The listing builds one solid part. Answer for the finished solid, in the listing's coordinates (mm). A direction names the side the tool comes from. Coordinates: 2 decimals unless noted, no trailing zeros. Loops run counter-clockwise (first coordinate to the right, second up) from the corner with the lowest first, then second, coordinate; pieces in that order, holes last. Notation, with made-up numbers: M -15.75,34 L 43.25,34 A27 cw 43.25,65 Z; hole C -35,84.5 d2. An arc over 180 degrees is marked long. Answer as a JSON object with one key per item and string values. Group by question number.
1. A cutting plane is placed at A-A on z = 62. Give the vertices of the cut face in (x, y).
2. Straight lines are drawn through the part: L1, parallel to X at y = -65, z = 36; L2, parallel to Y at x = -256.5, z = 40; L3, parallel to Z at x = -253.75, y = -165. For each, find the intervals that lie inside material, in ascending order.
3. For faces 4 (the face through (-262.797, -172.289, 94.33)), 5 (the face through (-262, -173, 88)), 6 (the face through (-262.4, -72.1, 76.9)), 7 (the face through (-247.6, -72.1, 76.9)), 8 (the face through (-255, -66, 50)), determine the directions among +Z, -Z, +X, -X, +Y, -Y from which every point of the face is accessible in a straight line to the end or side of a thin tool.
4. Given pin 1 (0.8 mm diameter, centred on y = -280, z = 109, fed in from -X); pin 2 (5 mm diameter, centred on x = -254.5, y = -283.5, fed in from -Z); pin 3 (3 mm diameter, centred on x = -249, y = -237.5, fed in from +Z); pin 4 (4 mm diameter, centred on x = -255, y = -285, fed in from +Z), each flat-ended and moving along its own axis, determine where each tip first touches the part or whether it passes through.
5. Determine the mould class of faces 1 (the face through (-248, -173, 88)), 2 (the face through (-254.93, -64.99, 25.61)), 3 (the face through (-246, -173, 89)) for opening direction X: released by +X, released by -X, zero draft, split by the parting line, or undercut.
from build123d import *

# Parameters (mm, degrees)
FORMED_WEB_DEPTH           = 10
EDGE_STIFFENING_LIPS_DEPTH = 206.123068282
WALL_MOUNT_HOLE_SKETCH_R   = 1.7
WALL_MOUNT_HOLES_DEPTH     = 2.4
COVER_MOUNT_HOLE_SKETCH_R  = 1.7
COVER_MOUNT_HOLE_DEPTH     = 2.4
LOWER_EDGE_CLEARANCE_DEPTH = 2.4


with BuildPart() as part:
    # Formed Web Section Sketch → Formed Web (new body)
    with BuildSketch(Plane(origin=(-260, 0, 0), x_dir=(0, 0, -1), z_dir=(1, 0, 0))):
        with BuildLine():
            Line((-22, -64), (-77.377483747, -64))
            ThreePointArc((-77.377483747, -64), (-80.010089753, -64.988457933), (-81.341585612, -67.46530719))
            Line((-81.341585612, -67.46530719), (-109.964101865, -279.66672079))
            ThreePointArc((-109.964101865, -279.66672079), (-109.991015376, -279.933465342), (-110, -280.2014136))
            Line((-110, -280.2014136), (-110, -290))
            Line((-110, -290), (-108, -290))
            Line((-108, -290), (-108, -280.2014136))
            ThreePointArc((-108, -280.2014136), (-107.995507688, -280.067439471), (-107.982050933, -279.934067195))
            Line((-107.982050933, -279.934067195), (-79.35953468, -67.732653595))
            ThreePointArc((-79.35953468, -67.732653595), (-78.69378675, -66.494228967), (-77.377483747, -66))
            Line((-77.377483747, -66), (-22, -66))
            Line((-22, -66), (-22, -64))
        make_face()
    extrude(amount=FORMED_WEB_DEPTH)

    # Edge Lip Sketch → Edge Stiffening Lips (add)
    with BuildSketch(Plane(origin=(0, -80.999511953, 10.925515566), x_dir=(-1, 0, 0), z_dir=(0, -0.9910254663478989, 0.1336732024376229))):
        with BuildLine():
            Line((264, -67.593279149), (264, -61.593279149))
            Line((264, -61.593279149), (262, -61.593279149))
            Line((262, -61.593279149), (262, -67.593279149))
            ThreePointArc((262, -67.593279149), (261.414213562, -69.007492712), (260, -69.593279149))
            Line((260, -69.593279149), (259.9, -69.593279149))
            Line((259.9, -69.593279149), (259.9, -71.593279149))
            Line((259.9, -71.593279149), (260, -71.593279149))
            ThreePointArc((260, -71.593279149), (262.828427125, -70.421706274), (264, -67.593279149))
        make_face()
        with BuildLine():
            Line((246, -67.593279149), (246, -61.593279149))
            Line((246, -61.593279149), (248, -61.593279149))
            Line((248, -61.593279149), (248, -67.593279149))
            ThreePointArc((248, -67.593279149), (248.585786438, -69.007492712), (250, -69.593279149))
            Line((250, -69.593279149), (250.1, -69.593279149))
            Line((250.1, -69.593279149), (250.1, -71.593279149))
            Line((250.1, -71.593279149), (250, -71.593279149))
            ThreePointArc((250, -71.593279149), (247.171572875, -70.421706274), (246, -67.593279149))
        make_face()
    extrude(amount=EDGE_STIFFENING_LIPS_DEPTH)

    # Wall Mount Hole Sketch → Wall Mount Holes (cut)
    with BuildSketch(Plane(origin=(0, -63.8, 0), x_dir=(-1, 0, 0), z_dir=(0, -1, 0))):
        with Locations(Location((255, -29, 0), (0, 0, 270))):
            Circle(WALL_MOUNT_HOLE_SKETCH_R)
        with Locations(Location((255, -36, 0), (0, 0, 270))):
            Circle(WALL_MOUNT_HOLE_SKETCH_R)
    extrude(amount=WALL_MOUNT_HOLES_DEPTH, mode=Mode.SUBTRACT)

    # Cover Mount Hole Sketch → Cover Mount Hole (cut)
    with BuildSketch(Plane.XY.offset(107.8)):
        with Locations(Location((-255, -285, 0), (0, 0, 90))):
            Circle(COVER_MOUNT_HOLE_SKETCH_R)
    extrude(amount=COVER_MOUNT_HOLE_DEPTH, mode=Mode.SUBTRACT)

    # Lower Edge Clearance Sketch → Lower Edge Clearance (cut)
    with BuildSketch(Plane(origin=(0, -63.8, 0), x_dir=(-1, 0, 0), z_dir=(0, -1, 0))):
        Polygon((261, -20), (249, -20), (249, -22.23), (261, -29.07), align=None)
    extrude(amount=LOWER_EDGE_CLEARANCE_DEPTH, mode=Mode.SUBTRACT)


solid = part.part
From the geometry:
{
 "1": {"outline": "M -260,-66 L -250,-66 L -250,-64 L -260,-64 Z"},
 "2": {"L1": "x = -260 to -256.7, -253.3 to -250", "L2": "y = -66 to -64", "L3": "z = 92.48 to 94.5"},
 "3": {"face 4": "+Z, -X, +Y", "face 5": "-Z, -Y", "face 6": "-Z, -X, +Y", "face 7": "-Z, +X, +Y", "face 8": "-Z, +X, -X, -Y"},
 "4": {"pin 1": "stops at x = -260", "pin 2": "stops at z = 108", "pin 3": "stops at z = 104.44", "pin 4": "stops at z = 110"},
 "5": {"face 1": "undercut", "face 2": "released by -X", "face 3": "released by +X"}
}
